Check sheet for the modelled part. Datum: model origin and axes. Units: mm. Face numbers are marked on the shaded views. A direction names the side the tool comes from. Round coordinates to 2 decimals unless told otherwise and drop trailing zeros. Order: outer loops, then holes, each group sorted by start corner. A loop starts at its lowest first (then second) coordinate and runs counter-clockwise, first axis right, second up. Notation, with made-up numbers: (-6, 18.5) -> (35, 18.5) arc R11 cw to (35, 33.5) -> close; hole circle Ø7 at (79, -1.75). An arc over 180 degrees is marked (long way). Answer in a Markdown table with one row per item.
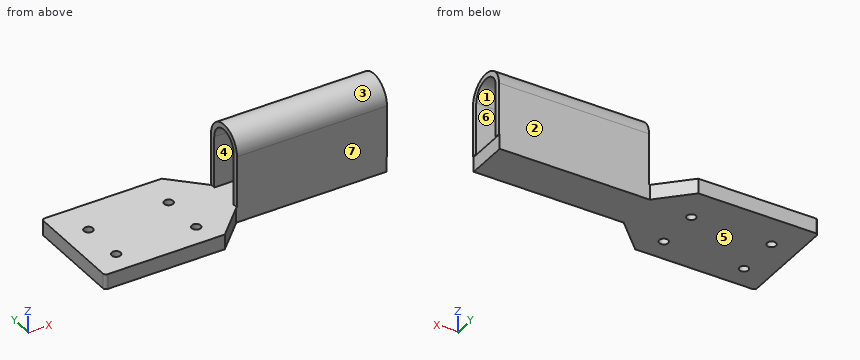
Autodesk Inventor part; units mm, degrees
ref_plane "Work Plane1" through (192, 0, 0) normal (1, 0, 0) x (0, 1, 0)
ref_plane "XZ Plane" through (0, 0, 0) normal (0, 1, 0) x (-1, 0, 0)
ref_plane "XY Plane" through (0, 0, 0) normal (0, 0, 1) x (1, 0, 0)
sketch "Sketch4" plane through (0, 0, 0) normal (0, 0, 1) x (1, 0, 0)
  line L0 (-8.4948, -28.1443) -> (-8.4948, 35.8557)
  line L1 (-6.4948, 37.8557) -> (71.5052, 37.8557)
  line L2 (71.5052, 37.8557) -> (91.5052, 17.8557)
  line L3 (-6.4948, -30.1443) -> (71.5052, -30.1443)
  line L4 (71.5052, -30.1443) -> (91.5052, -10.1443)
  line L5 (91.5052, -10.1443) -> (91.5052, 17.8557)
  line L6 (91.5052, 17.8557) -> (191.5052, 17.8557)
  line L7 (191.5052, 17.8557) -> (191.5052, -10.1443)
  line L8 (191.5052, -10.1443) -> (91.5052, -10.1443)
  arc A0 (-6.4948, 37.8557) -> (-8.4948, 35.8557) centre (-6.4948, 35.8557) ccw
  arc A1 (-8.4948, -28.1443) -> (-6.4948, -30.1443) centre (-6.4948, -28.1443) ccw
  line L9 (71.5052, 37.8557) -> (91.5052, 17.8557)
  line L10 (71.5052, -30.1443) -> (91.5052, -10.1443)
  line L11 (91.5052, 17.8557) -> (91.5052, -10.1443)
  point P0 (0, 0)
  point P1 (-8.4948, -30.1443)
  point P2 (-8.4948, 37.8557)
  dimension "d7" = 68
  dimension "d8" = 80
  dimension "d9" = 80
  dimension "d10" = 135
  dimension "d11" = 135
  dimension "d12" = 20
  dimension "d13" = 20
  dimension "d14" = 28
  dimension "d15" = 2
  dimension "d16" = 2
  dimension "d19" = 100
extrude "Extrusion2" add sketch "Sketch4" along normal blind 10
ref_plane "Work Plane1" through (192, 0, 0) normal (1, 0, 0) x (0, 1, 0)
sketch "Sketch5" plane through (192, 0, 0) normal (1, 0, 0) x (0, 1, 0)
  line L0 (17.8557, 10) -> (17.8557, 44.45)
  line L1 (-10.1443, 0) -> (-10.1443, 10)
  line L2 (-10.1443, 10) -> (-10.1443, 44.45)
  arc A0 (17.8557, 44.45) -> (-10.1443, 44.45) centre (3.8557, 44.45) ccw
  line L3 (14.3557, 10) -> (14.3557, 44.45)
  line L4 (-6.6443, 10) -> (-6.6443, 44.45)
  arc A1 (14.3557, 44.45) -> (-6.6443, 44.45) centre (3.8557, 44.45) ccw
  line L5 (14.3557, 44.45) -> (14.3557, 10)
  line L6 (-6.6443, 44.45) -> (-6.6443, 10)
  line L7 (-10.1443, 10) -> (17.8557, 10)
  line L8 (17.8557, 10) -> (14.3557, 10)
  line L9 (-6.6443, 10) -> (-10.1443, 10)
  point P0 (0, 0)
  dimension "d21" = 34.45
  dimension "d22" = 3.5
  dimension "d23" = 3.5
extrude "Extrusion3" add sketch "Sketch5" against normal blind 100 contours L7 L3 A1 L4 L2 A0 L0
sketch "Sketch6" plane through (0, 0, 0) normal (0, 0, 1) x (1, 0, 0)
  line L0 (-54.1714, 0) -> (81.2571, 0)
  line L1 (8.4643, 0) -> (8.4643, 14.85)
  line L2 (8.4643, 0) -> (8.4643, -14.85)
  circle A0 centre (8.4643, 14.85) radius 3
  circle A1 centre (8.4643, -14.85) radius 3
  line L3 (61.9125, 0) -> (61.9125, 14.85)
  line L4 (61.9125, 0) -> (61.9125, -14.85)
  circle A2 centre (61.9125, 14.85) radius 3
  circle A3 centre (61.9125, -14.85) radius 3
  point P0 (0, 0)
  dimension "d26" = 14.85
  dimension "d27" = 14.85
  dimension "d28" = 6
  dimension "d29" = 6
  dimension "d30" = 14.85
  dimension "d31" = 14.85
  dimension "d32" = 6
  dimension "d33" = 6
extrude "Extrusion4" cut sketch "Sketch6" along normal blind 10
thread "Thread1"
thread "Thread2"
thread "Thread3"
thread "Thread4"
properties part number "WireHolderPiece1"
Item 1: Set-up check for the marked faces 1, 2 and 3: record each of +Z, -Z, +X, -X, +Y, -Y from which the full face is reachable in a straight line by a thin tool's end or side.
Result sheet:
| item | result |
|---|---|
| face 1 | +X, -X |
| face 2 | +Z, -Z, +X, +Y |
| face 3 | +Z, +X, -X |
Item 2: Cross-section at C-C (x = 50). Record the boundary of the cut face in (y, z), and give its area (3 significant figures).
Result sheet:
| item | result |
|---|---|
| outline | (-30.14, 0) -> (37.86, 0) -> (37.86, 10) -> (-30.14, 10) -> close |
| area | 680 mm^2 |
Item 3: Mould release check, pull along Y, two halves, no side actions. Record for the marked faces 4, 5, 6 and 7: pulls with the +Y half, pulls with the -Y half, needs draft (parallel to the pull), parting line crosses it, or undercut.
Result sheet:
| item | result |
|---|---|
| face 4 | undercut |
| face 5 | needs draft |
| face 6 | undercut |
| face 7 | pulls with the -Y half |
Item 4: Scan lines: line 1 (Y direction, x = 117, z = 41); line 2 (X direction, y = 14.85, z = 6.5); line 3 (X direction, y = -14, z = 6). Record each from-to range of solid material in increasing order. Write a range as [from, to].
Result sheet:
| item | result |
|---|---|
| line 1 | y = [-10.14, -6.64], [14.36, 17.86] |
| line 2 | x = [-8.49, 5.46], [11.46, 58.91], [64.91, 191.51] |
| line 3 | x = [-8.49, 5.59], [11.34, 59.04], [64.79, 87.65] |
Item 5: Cross-section at A-A (z = 21). Record the boundary of the cut face in (x, y), and give its area (3 significant figures).
Result sheet:
| item | result |
|---|---|
| outline | (92, -10.14) -> (192, -10.14) -> (192, -6.64) -> (92, -6.64) -> close; (92, 14.36) -> (192, 14.36) -> (192, 17.86) -> (92, 17.86) -> close |
| area | 700 mm^2 |
Item 6: Cross-section at B-B (y = -14.85). Record the boundary of the cut face in (x, z), and give its area (3 significant figures).
Result sheet:
| item | result |
|---|---|
| outline | (-8.49, 0) -> (5.46, 0) -> (5.46, 10) -> (-8.49, 10) -> close; (11.46, 0) -> (58.91, 0) -> (58.91, 10) -> (11.46, 10) -> close; (64.91, 0) -> (86.8, 0) -> (86.8, 10) -> (64.91, 10) -> close |
| area | 833 mm^2 |
Item 7: Cross-section at D-D (z = 53). Record the boundary of the cut face in (x, y).
Result sheet:
| item | result |
|---|---|
| outline | (92, -7.23) -> (192, -7.23) -> (192, -2.24) -> (92, -2.24) -> close; (92, 9.95) -> (192, 9.95) -> (192, 14.94) -> (92, 14.94) -> close |
Item 8: Depth check by flat-ended pin: P1, Ø0.5, axis at x = 192, y = 16.5, coming from the -Z side; P2, Ø3, axis at y = 13.5, z = 31.5, coming from the -X side; P3, Ø10, axis at x = 139, y = -12, coming from the +Z side. Enter the tip coordinate at first touch or a pass-through.
Result sheet:
| item | result |
|---|---|
| P1 | stops at z = 10 |
| P2 | stops at x = 92 |
| P3 | stops at z = 53.29 |
